Can you work these out from the drawing? Everything is in mm from the part's minimum corner. A direction names the side the tool comes from. Give positions to 0.01 mm unless a question says otherwise; leave off trailing zeros. Write each loop counter-clockwise with the first axis right and the second up, starting at its lowest first coordinate (ties: lowest second). Pieces come first, ordered by that corner, then holes. Notation, with made-up numbers: (77, 16) - (100, 16) arc R5 cw to (100, 22) - close; hole circle Ø11 at (80, 76). An arc over 180 degrees is marked (long way). Use a Markdown table: item, result.
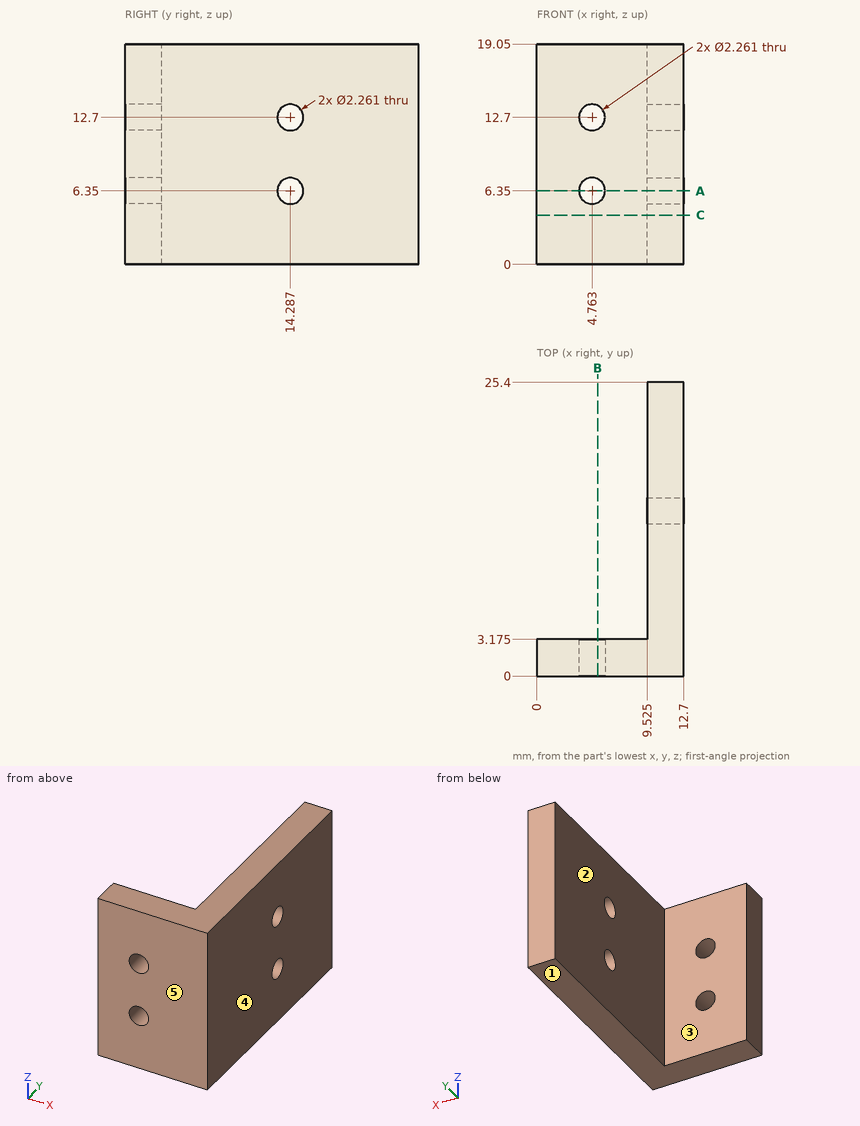
Item 1: Thinking about a two-plate mould opening in Y: for the marked faces 3, 4 and 5, which applies, +Y half, -Y half, draft (parallel to the pull), parting line (faces both ways), or undercut?
Values:
| item | result |
|---|---|
| face 3 | +Y half |
| face 4 | draft |
| face 5 | -Y half |
Item 2: Will these pins go through, and if not, where does the flat tip stop? pin 1 Ø2.5 at (x, z) = (4.76, 12.7) entering from -Y; pin 2 Ø3.5 at (x, z) = (4.76, 6.35) entering from +Y (1 decimal); pin 3 Ø3.5 at (y, z) = (14.29, 6.35) entering from -X (1 decimal).
Values:
| item | result |
|---|---|
| pin 1 | stops at y = 0 |
| pin 2 | stops at y = 3.2 |
| pin 3 | stops at x = 9.5 |
Item 3: I need wall thicknesses on line 1 along X through (y, z) = (2.1, 12.7); line 2 along Y through (x, z) = (11.1, 6.35); line 3 along X through (y, z) = (22.5, 10) (1 decimal). Which ranges of each line are inside material? Lowest first, please. Write a range as [from, to].
Values:
| item | result |
|---|---|
| line 1 | x = [0, 3.63], [5.89, 12.7] |
| line 2 | y = [0, 13.16], [15.42, 25.4] |
| line 3 | x = [9.5, 12.7] |
Item 4: If we section it at A-A, the plane z = 6.35: Write out the boundary of the cut face in (x, y) (1 decimal).
Values:
| item | result |
|---|---|
| outline | (0, 0) - (3.6, 0) - (3.6, 3.2) - (0, 3.2) - close; (5.9, 0) - (12.7, 0) - (12.7, 13.2) - (9.5, 13.2) - (9.5, 3.2) - (5.9, 3.2) - close; (9.5, 15.4) - (12.7, 15.4) - (12.7, 25.4) - (9.5, 25.4) - close |
Item 5: If we section it at B-B, the plane x = 5.25: Count the separate pieces of the cut face and the enclosed holes in it.
Values:
| item | result |
|---|---|
| separate pieces | 3 |
| enclosed holes | 0 |
Item 6: If we section it at C-C, the plane z = 4.25: Write out the boundary of the cut face in (x, y) (1 decimal), plus the area to 3 significant figures.
Values:
| item | result |
|---|---|
| outline | (0, 0) - (12.7, 0) - (12.7, 25.4) - (9.5, 25.4) - (9.5, 3.2) - (0, 3.2) - close |
| area | 111 mm2 |
Item 7: For the marked faces 1 and 2, which set-ups out of +Z, -Z, +X, -X, +Y, -Y let a thin tool reach every point of the face, with its end or its side?
Values:
| item | result |
|---|---|
| face 1 | -Z, +X, -X, +Y, -Y |
| face 2 | +Z, -Z, -X, +Y |
